Work out the finished part from the listing and answer in its coordinate system (mm). Coordinates: 2 decimals unless noted, no trailing zeros. Order: outer loops, then holes, each group sorted by start corner. A loop starts at its lowest first (then second) coordinate and runs counter-clockwise, first axis right, second up. Notation, with made-up numbers: (76, 4.5) -> (114, 4.5) arc R33 ccw to (114, 36.5) -> close; hole circle Ø8 at (-8.75, 77.5). An arc over 180 degrees is marked (long way). Answer as CSV lines item,"result". Start each with the question number.
Item 1: Section A-A (x = 10.5) is taken. Write down the section's boundary in (y, z), then the cut area to 3 significant figures.
Item 2: Section B-B (z = -10) is taken. Write down the section's boundary in (x, y), then the cut area to 3 significant figures.
Item 3: Straight lines are drawn through the part: L1, parallel to X at y = 24, z = 0; L2, parallel to Z at x = -16, y = 32.5. For each, find the intervals that lie inside material, in ascending order.
Item 4: Each of these flat-tipped pins is pushed along its axis until it touches: pin 1 Ø5 at (x, z) = (0, 0) entering from -Y; pin 2 Ø4 at (x, y) = (1.5, 170) entering from +Z; pin 3 Ø7.5 at (x, y) = (0, 58) entering from -Z. Where does it stop, or does it pass through?
```python
from build123d import *

# Parameters (mm, degrees)
EXTRUDE1_DEPTH = 230.9876


# Read off the part's stored shape, not the designer's step: 1515<1>
with BuildPart() as part:
    # Sketch1<2> → Extrude1 (new body)
    with BuildSketch(Plane(origin=(0, 0, 0), x_dir=(1, 0, 0), z_dir=(0, 1, 0))):
        Polygon((-6.7564, 4.364749804), (-6.7564, -4.364749804), (-14.986, -12.594349804), (-14.986, -4.064), (-19.05, -4.064), (-19.05, -19.05), (-4.064, -19.05), (-4.064, -14.986), (-13.067127258, -14.986), (-4.837527258, -6.7564), (4.837527258, -6.7564), (13.067127258, -14.986), (4.064, -14.986), (4.064, -19.05), (19.05, -19.05), (19.05, -4.064), (14.986, -4.064), (14.986, -12.594349804), (6.7564, -4.364749804), (6.7564, 4.364749804), (14.986, 12.594349804), (14.986, 4.064), (19.05, 4.064), (19.05, 19.05), (4.064, 19.05), (4.064, 14.986), (13.067127258, 14.986), (4.837527258, 6.7564), (-4.837527258, 6.7564), (-13.067127258, 14.986), (-4.064, 14.986), (-4.064, 19.05), (-19.05, 19.05), (-19.05, 4.064), (-14.986, 4.064), (-14.986, 12.594349804), align=None)
    extrude(amount=EXTRUDE1_DEPTH)

    # Sketch2 → 5/16-18 Tapped Hole1 (revolve, cut)
    with BuildSketch(Plane(origin=(0, 230.9876, 0), x_dir=(0, 0, 1), z_dir=(1, 0, 0))):
        Polygon((0, 0), (0, 33.711148974), (3.2639, 31.75), (3.2639, 0), align=None)
    f_5_16_18_tapped_hole1 = revolve(axis=Axis((0, 237.3376, 0), (0, -1, 0)), mode=Mode.SUBTRACT)

    # Mirror1: 5/16-18 Tapped Hole1 across plane
    add(f_5_16_18_tapped_hole1.mirror(Plane.ZX.offset(115.4938)), mode=Mode.SUBTRACT)


solid = part.part
```
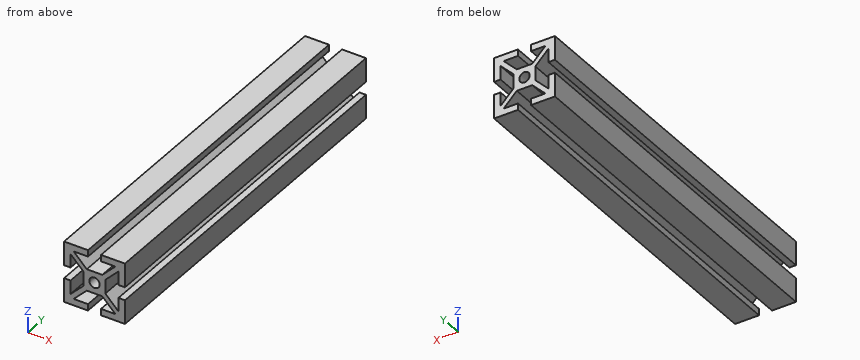
Checked values:
1,outline,"(0, -19.05) -> (230.99, -19.05) -> (230.99, -14.99) -> (0, -14.99) -> close; (0, -12.42) -> (230.99, -12.42) -> (230.99, -8.11) -> (0, -8.11) -> close; (0, 8.11) -> (230.99, 8.11) -> (230.99, 12.42) -> (0, 12.42) -> close; (0, 14.99) -> (230.99, 14.99) -> (230.99, 19.05) -> (0, 19.05) -> close"
1,area,"3,870 mm^2"
2,outline,"(-19.05, 0) -> (-14.99, 0) -> (-14.99, 230.99) -> (-19.05, 230.99) -> close; (-12.39, 0) -> (-8.08, 0) -> (-8.08, 230.99) -> (-12.39, 230.99) -> close; (8.08, 0) -> (12.39, 0) -> (12.39, 230.99) -> (8.08, 230.99) -> close; (14.99, 0) -> (19.05, 0) -> (19.05, 230.99) -> (14.99, 230.99) -> close"
2,area,"3,870 mm^2"
3,L1,"x = -6.76 to -3.26, 3.26 to 6.76"
3,L2,"z = -19.05 to -4.06, 4.06 to 19.05"
4,pin 1,"stops at y = 32.21"
4,pin 2,"stops at z = 6.76"
4,pin 3,"stops at z = -6.76"
